For this review, take the finished solid that the model builds, in its own axes (mm). Face numbers are marked on the shaded views. A direction names the side the tool comes from. Give positions to 0.01 mm unless a question says otherwise; leave off trailing zeros. Loops run counter-clockwise (first coordinate to the right, second up) from the corner with the lowest first, then second, coordinate; pieces in that order, holes last. Notation, with made-up numbers: (73.25, 40.5) -> (112.25, 40.5) arc R35 ccw to (112.25, 72.5) -> close; hole circle Ø3 at (74, 18). An arc over 180 degrees is marked (long way). One line per question, with ' | ' between items. Start each with the question number.
(1) Insertion check: P1, Ø4, axis at x = 20, y = -0.5, coming from the +Z side; P2, Ø5, axis at x = 9, z = 4, coming from the +Y side; P3, Ø13, axis at x = -1.5, z = 15.5, coming from the -Y side; P4, Ø4, axis at y = -17, z = 10.5, coming from the -X side. Each pin has a flat end and moves straight along its axis. Give the tip position at first contact, or say it passes through.
(2) Consider section A-A (y = 0). Write out the cut boundary in (x, z).
(3) Tool access review of the marked faces 1, 2 and 3: name each direction out of +Z, -Z, +X, -X, +Y, -Y from which nothing blocks a thin tool from reaching the whole face with its end or side.
(4) Consider section D-D (x = 16). Write out the cut boundary in (y, z), and give its area (3 significant figures).
(5) Consider section B-B (x = 0). Write out the cut boundary in (y, z), and give its area (3 significant figures).
(6) Consider section C-C (z = 12). Write out the cut boundary in (x, y) (3 decimals), and give its area (3 significant figures).
(7) Draft analysis for pull direction Y (two halves, no side actions). For the marked faces 4, 5 and 6, state which applies: +Y half, -Y half, draft (parallel to the pull), parting line (faces both ways), or undercut.
(8) Wall thickness on probe 1 along Y at (x, z) = (-9, 17.5); probe 2 along Y at (x, z) = (19, 9); probe 3 along X at (y, z) = (-17, 2.75): over which ranges is each line inside the solid? List them lowest first.
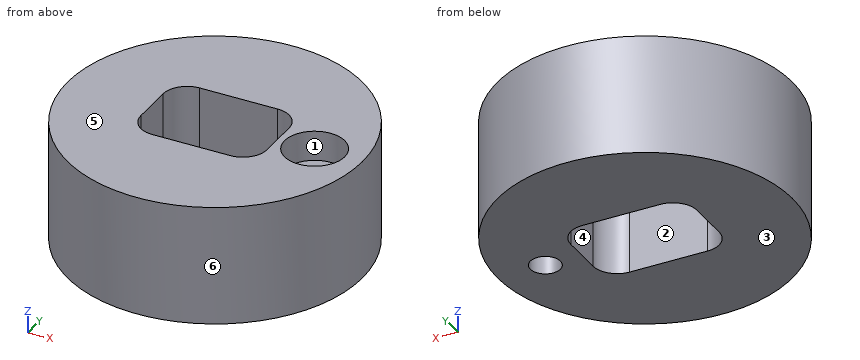
from build123d import *

# Parameters (mm, degrees)
F0_R           = 31.109261
F1_DEPTH       = 25.4
F2_W           = 26.62818
F2_H           = 19.062922
F3_DEPTH       = 25.4
F4_R           = 5.08
F6_D           = 6.35
F6_CBORE_D     = 12.7
F6_CBORE_DEPTH = 6.35


with BuildPart() as f1:
    # F0 (on Top) → F1 (new body)
    with BuildSketch(Plane.XY):
        Circle(F0_R)
    extrude(amount=F1_DEPTH)

    # F2 (on face) → F3 (cut)
    with BuildSketch(Plane.XY.offset(25.4)):
        Rectangle(F2_W, F2_H)
    extrude(amount=-F3_DEPTH, mode=Mode.SUBTRACT)

    # F4
    f4_edges = [f1.edges().sort_by_distance(p)[0] for p in [
        (-13.31409, 9.531461, 12.7),
        (-13.31409, -9.531461, 12.7),
        (13.31409, 9.531461, 12.7),
        (13.31409, -9.531461, 12.7),
    ]]
    fillet(f4_edges, radius=F4_R)

    # F6 (through all)
    with Locations(Plane.XY.offset(25.4)):
        with Locations((21.028863, 0)):
            CounterBoreHole(F6_D / 2, F6_CBORE_D / 2, F6_CBORE_DEPTH)


solid = f1.part
A:
1) P1: passes through | P2: stops at y = 30.42 | P3: stops at y = -31.11 | P4: stops at x = -27.25
2) outline: (-31.11, 0) -> (-13.31, 0) -> (-13.31, 25.4) -> (-31.11, 25.4) -> close; (13.31, 0) -> (17.85, 0) -> (17.85, 19.05) -> (14.68, 19.05) -> (14.68, 25.4) -> (13.31, 25.4) -> close; (24.2, 0) -> (31.11, 0) -> (31.11, 25.4) -> (27.38, 25.4) -> (27.38, 19.05) -> (24.2, 19.05) -> close
3) face 1: +Z | face 2: +Z, -Z | face 3: -Z, +X, -X, +Y, -Y
4) outline: (-26.68, 0) -> (26.68, 0) -> (26.68, 25.4) -> (3.88, 25.4) -> (3.88, 19.05) -> (-3.88, 19.05) -> (-3.88, 25.4) -> (-26.68, 25.4) -> close | area: 1,310 mm^2
5) outline: (-31.11, 0) -> (-9.53, 0) -> (-9.53, 25.4) -> (-31.11, 25.4) -> close; (9.53, 0) -> (31.11, 0) -> (31.11, 25.4) -> (9.53, 25.4) -> close | area: 1,100 mm^2
6) outline: circle Ø62.219 at (0, 0); hole (-13.314, -4.451) arc R5.08 ccw to (-8.234, -9.531) -> (8.234, -9.531) arc R5.08 ccw to (13.314, -4.451) -> (13.314, 4.451) arc R5.08 ccw to (8.234, 9.531) -> (-8.234, 9.531) arc R5.08 ccw to (-13.314, 4.451) -> close; hole circle Ø6.35 at (21.029, 0) | area: 2,520 mm^2
7) face 4: undercut | face 5: draft | face 6: parting line
8) probe 1: y = -29.78 to -9.47, 9.47 to 29.78 | probe 2: y = -24.63 to -2.44, 2.44 to 24.63 | probe 3: x = -26.05 to 26.05
